The listing builds one solid part. Answer for the finished solid, in the listing's coordinates (mm). Face numbers are marked on the shaded views. A direction names the side the tool comes from. Give positions to 0.01 mm unless a question says otherwise; leave off trailing zeros. Loops run counter-clockwise (first coordinate to the right, second up) from the corner with the lowest first, then second, coordinate; pieces in that order, holes last. Notation, with made-up numbers: (39, 36.25) - (73, 36.25) arc R31 cw to (73, 72.25) - close; hole circle Ø7 at (46.25, -39). An arc over 180 degrees is marked (long way). Write each question's results on one line, items separated by ' | '.
from build123d import *

# Parameters (mm, degrees)
F1_DEPTH = 25.4
F2_SIZE  = 5
F3_R     = 6
F4_W     = 12
F4_H     = 5
F5_DEPTH = 25
F6_R     = 5
F7_R     = 10
F8_DEPTH = 25
F9_R     = 7.5


with BuildPart() as f1:
    # F0 (on Front) → F1 (new body)
    with BuildSketch(Plane.XZ):
        Polygon((43.3064028621, 0), (0, 29.9521442503), (-43.4733256698, 0), (0, -22.7049794048), align=None)
    extrude(amount=F1_DEPTH)

    # F2
    f2_edges = [f1.edges().sort_by_distance(p)[0] for p in [
        (-21.736663, 0, 14.976072),
        (-21.736663, 0, -11.35249),
        (21.653201, 0, -11.35249),
        (21.653201, 0, 14.976072),
    ]]
    chamfer(f2_edges, length=F2_SIZE)

    # F3
    f3_edges = [f1.edges().sort_by_distance(p)[0] for p in [
        (-21.736663, -25.4, 14.976072),
        (21.653201, -25.4, 14.976072),
        (21.653201, -25.4, -11.35249),
        (-21.736663, -25.4, -11.35249),
    ]]
    fillet(f3_edges, radius=F3_R)

    # F4 (on face) → F5 (cut)
    with BuildSketch(Plane(origin=(-13.9936893699, 0, 20.3108068062), x_dir=(0.8234735009, 0, 0.5673547332), z_dir=(-0.5673547332, 0, 0.8234735009))):
        with Locations((0.9934908095, -12.9)):
            Rectangle(F4_W, F4_H)
    extrude(amount=-F5_DEPTH, mode=Mode.SUBTRACT)

    # F6
    f6_edges = [f1.edges().sort_by_distance(p)[0] for p in [
        (-16.903935, 0, -8.235641),
        (16.829559, 0, -8.23594),
    ]]
    fillet(f6_edges, radius=F6_R)

    # F7 (on face) → F8 (join)
    with BuildSketch(Plane.XZ.offset(25.4)):
        with Locations((0.3409804194, 2.2267708555)):
            Circle(F7_R)
    extrude(amount=F8_DEPTH)

    # F9
    f9_edges = [f1.edges().sort_by_distance(p)[0] for p in [
        (-9.65902, -50.4, 2.226771),
    ]]
    fillet(f9_edges, radius=F9_R)


solid = f1.part
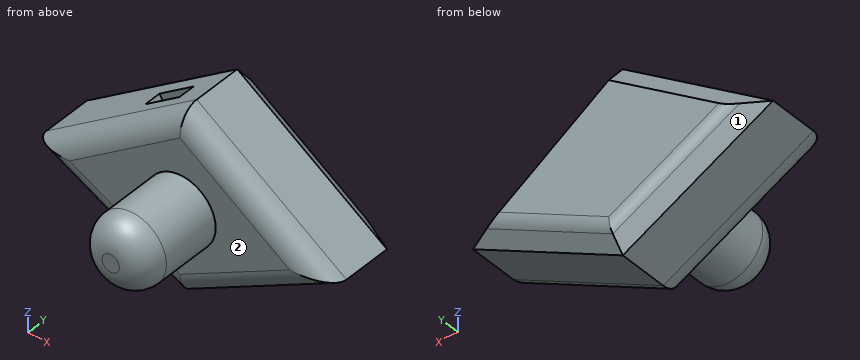
Item 1: A cutting plane is placed at C-C, the plane y = -33.5. Determine the outline of the cut face in (x, z), plus the area to 3 significant figures.
Values found:
outline: circle Ø20 at (0.34, 2.23) | area: 314 mm²
Item 2: A cutting plane is placed at A-A, the plane y = -12. Determine the outline of the cut face in (x, z), plus the area to 3 significant figures.
Values found:
outline: (-43.47, 0) - (0, -22.7) - (43.31, 0) - (0, 29.95) - (-8.23, 24.28) - (5.95, 3.69) - (-3.93, -3.12) - (-18.12, 17.47) - close | area: 1,980 mm²
Item 3: A cutting plane is placed at B-B, the plane y = -4. Determine the outline of the cut face in (x, z), plus the area to 3 significant figures.
Values found:
outline: (-41.54, 0.12) - (0, -21.58) - (41.38, 0.12) - (0, 28.74) - close | area: 2,090 mm²
Item 4: Find the intervals of material crossed by line 1 along Y through (x, z) = (-2.5, 14.5); line 2 along Y through (x, z) = (1.5, -14.5); line 3 along X through (y, z) = (-11.5, 10.5), in increasing order. Write a range as [from, to].
Values found:
line 1: y = [-25.4, -15.4], [-10.4, 0] | line 2: y = [-25.4, -0.03] | line 3: x = [-28.23, -13.31], [1.26, 28.12]
Item 5: Flat-ended cylindrical pins translate along their axes: P1, Ø6, axis at y = -34, z = 17.5, coming from the +X side; P2, Ø12, axis at x = 4.5, y = -44, coming from the -Z side; P3, Ø8, axis at x = -33.5, z = 1.5, coming from the -Y side; P4, Ø7, axis at x = -5, z = 10.5, coming from the -Y side. Find the tip coordinate at first contact, or state that the pin passes through.
Values found:
P1: passes through | P2: stops at z = -7.77 | P3: stops at y = -25.4 | P4: stops at y = -49.34
Item 6: For the marked faces 1 and 2, determine the directions among +Z, -Z, +X, -X, +Y, -Y from which every point of the face is accessible in a straight line to the end or side of a thin tool.
Values found:
face 1: -Z, -X, +Y | face 2: -Y
